from build123d import *

# Parameters (mm, degrees)
F0_W         = 15
F0_H         = 160
F0_R         = 1.55
F1_DEPTH     = 5
F2_R         = 5
F3_T1_DEPTH  = 150
F3_T3_DEPTH  = 5
F3_T6_ANGLE  = 90
F3_T8_ANGLE  = 90
F3_T10_ANGLE = 90
F3_T12_ANGLE = 90


# Not quite as in the source:
# - a fillet or chamfer that OpenCascade refuses, or shapes differently, is made with other operations: its cross-section is extruded or revolved along the edge and cut away or added


with BuildPart() as f1:
    # F0 (on Top) → F1 (new body)
    with BuildSketch(Plane.XY):
        Rectangle(F0_W, F0_H)
        with Locations((-5, -75)):
            Circle(F0_R, mode=Mode.SUBTRACT)
        with BuildLine():
            ThreePointArc((6.55, -75), (5, -76.55), (3.45, -75))
            ThreePointArc((3.45, -75), (5, -73.45), (6.55, -75))
        make_face(mode=Mode.SUBTRACT)
        with Locations((-5, 75)):
            Circle(F0_R, mode=Mode.SUBTRACT)
        with BuildLine():
            ThreePointArc((6.55, 75), (5, 73.45), (3.45, 75))
            ThreePointArc((3.45, 75), (5, 76.55), (6.55, 75))
        make_face(mode=Mode.SUBTRACT)
    extrude(amount=F1_DEPTH)

    # F2
    f2_edges = [f1.edges().sort_by_distance(p)[0] for p in [
        (7.5, -80, 2.5),
        (-7.5, -80, 2.5),
        (7.5, 80, 2.5),
        (-7.5, 80, 2.5),
    ]]
    fillet(f2_edges, radius=F2_R)

    # F3: fillet of radius 1 on 8 edges, made by hand

    # F3_s2 → F3_t1 (cut)
    with BuildSketch(Plane.XZ.offset(-75)):
        with BuildLine():
            ThreePointArc((6.5, 5), (7.2071067812, 4.7071067812), (7.5, 4))
            Line((7.5, 4), (7.5, 5))
            Line((7.5, 5), (6.5, 5))
        make_face()
        with BuildLine():
            ThreePointArc((-7.5, 4), (-7.2071067812, 4.7071067812), (-6.5, 5))
            Line((-6.5, 5), (-7.5, 5))
            Line((-7.5, 5), (-7.5, 4))
        make_face()
    extrude(amount=F3_T1_DEPTH, mode=Mode.SUBTRACT)

    # F3_s4 → F3_t3 (cut)
    with BuildSketch(Plane.YZ.offset(-2.5)):
        with BuildLine():
            ThreePointArc((79, 5), (79.7071067812, 4.7071067812), (80, 4))
            Line((80, 4), (80, 5))
            Line((80, 5), (79, 5))
        make_face()
        with BuildLine():
            ThreePointArc((-79, 5), (-79.7071067812, 4.7071067812), (-80, 4))
            Line((-80, 4), (-80, 5))
            Line((-80, 5), (-79, 5))
        make_face()
    extrude(amount=F3_T3_DEPTH, mode=Mode.SUBTRACT)

    # F3_s5 → F3_t6 (revolve, cut)
    with BuildSketch(Plane.XZ.offset(-75)):
        with BuildLine():
            ThreePointArc((-7.5, 4), (-7.2071067812, 4.7071067812), (-6.5, 5))
            Line((-6.5, 5), (-7.5, 5))
            Line((-7.5, 5), (-7.5, 4))
        make_face()
    revolve(axis=Axis((-2.5, 75, 5), (0, 0, -1)), revolution_arc=F3_T6_ANGLE, mode=Mode.SUBTRACT)

    # F3_s7 → F3_t8 (revolve, cut)
    with BuildSketch(Plane.XZ.offset(75)):
        with BuildLine():
            ThreePointArc((-7.5, 4), (-7.2071067812, 4.7071067812), (-6.5, 5))
            Line((-6.5, 5), (-7.5, 5))
            Line((-7.5, 5), (-7.5, 4))
        make_face()
    revolve(axis=Axis((-2.5, -75, 5), (0, 0, 1)), revolution_arc=F3_T8_ANGLE, mode=Mode.SUBTRACT)

    # F3_s9 → F3_t10 (revolve, cut)
    with BuildSketch(Plane.XZ.offset(-75)):
        with BuildLine():
            ThreePointArc((6.5, 5), (7.2071067812, 4.7071067812), (7.5, 4))
            Line((7.5, 4), (7.5, 5))
            Line((7.5, 5), (6.5, 5))
        make_face()
    revolve(axis=Axis((2.5, 75, 5), (0, 0, 1)), revolution_arc=F3_T10_ANGLE, mode=Mode.SUBTRACT)

    # F3_s11 → F3_t12 (revolve, cut)
    with BuildSketch(Plane.XZ.offset(75)):
        with BuildLine():
            ThreePointArc((6.5, 5), (7.2071067812, 4.7071067812), (7.5, 4))
            Line((7.5, 4), (7.5, 5))
            Line((7.5, 5), (6.5, 5))
        make_face()
    revolve(axis=Axis((2.5, -75, 5), (0, 0, -1)), revolution_arc=F3_T12_ANGLE, mode=Mode.SUBTRACT)


solid = f1.part
Build history of the part. All positions in model axes, mm. Round coordinates to 2 decimals unless told otherwise and drop trailing zeros. Loops run counter-clockwise (first coordinate to the right, second up) from the corner with the lowest first, then second, coordinate; pieces in that order, holes last. Notation, with made-up numbers: (10, 62) -> (36, 62) arc R24 ccw to (36, 78) -> close; hole circle Ø4 at (58, -33.75). An arc over 180 degrees is marked (long way). Use CSV: the item, a comma, the result in double quotes. Start each with the question number.
Q1. Drill centre lines: L1, parallel to X at y = -75, z = 1.75; L2, parallel to Y at x = -5, z = 2.3; L3, parallel to Y at x = -5.25, z = 4.2. Where is each one in solid material? Low to high.
Q2. Mould opens along X. For faces 1 (the face through (0, 1, 0)), 2 (the face through (6, -78.57, 2.03)), 3 (the face through (-6.07, -78.5, 2.03)), 4 (the face through (-5.202, -73.463, 2.465)) say: +X half, -X half, draft (parallel to the pull), parting line (faces both ways), or undercut.
Q3. Saw through at A-A on z = 1.1. Give the cut face in (x, y).
Q4. Flat gauge pins, fed straight in: pin 1 Ø1.5 at (x, z) = (5, 3) entering from -Y; pin 2 Ø8 at (x, y) = (2, -1.5) entering from -Z. Where does each tip first touch, or does it go through?
Q5. Saw through at B-B on x = -4.75. Count the separate pieces of the cut face and the enclosed holes in it, and give its area (3 significant figures).
Solutions:
1,L1,"x = -7.5 to -6.55, -3.45 to 3.45, 6.55 to 7.5"
1,L2,"y = -79.33 to -76.55, -73.45 to 73.45, 76.55 to 79.33"
1,L3,"y = -79.15 to -76.53, -73.47 to 73.47, 76.53 to 79.15"
2,face 1,"draft"
2,face 2,"+X half"
2,face 3,"-X half"
2,face 4,"undercut"
3,outline,"(-7.5, -75) arc R5 ccw to (-2.5, -80) -> (2.5, -80) arc R5 ccw to (7.5, -75) -> (7.5, 75) arc R5 ccw to (2.5, 80) -> (-2.5, 80) arc R5 ccw to (-7.5, 75) -> close; hole circle Ø3.1 at (-5, -75); hole circle Ø3.1 at (-5, 75); hole circle Ø3.1 at (5, -75); hole circle Ø3.1 at (5, 75)"
4,pin 1,"stops at y = -79.68"
4,pin 2,"stops at z = 0"
5,separate pieces,"3"
5,enclosed holes,"0"
5,area,"764 mm^2"
